Can you work these out from the model? Positions are in its coordinate system, mm. A direction names the side the tool comes from. Give positions to 0.01 mm unless a question says otherwise; leave off trailing zeros. Order: outer loops, then holes, each group sorted by start corner. A loop starts at its lowest first (then second) coordinate and runs counter-clockwise, first axis right, second up. Notation, with made-up numbers: (26, -7.75) - (49, -7.75) arc R26 cw to (49, 10.25) - close; hole circle Ø6 at (3.5, 58). An arc over 180 degrees is marked (long way). Answer as a JSON object with one key per item and string values.
```python
from build123d import *

# Parameters (mm, degrees)
BOSS_EXTRUDE1_DEPTH = 1.27


with BuildPart() as part:
    # Sketch1 → Boss-Extrude1 (new body)
    with BuildSketch(Plane(origin=(0, 0, 0), x_dir=(1, 0, 0), z_dir=(0, 1, 0))):
        with BuildLine():
            Line((-152.4, 120.65), (-139.7, -120.65))
            Line((-139.7, -120.65), (-134.247237287, -224.252491542))
            ThreePointArc((-134.247237287, -224.252491542), (-122.423123118, -249.88969001), (-96.19989799, -260.35))
            Line((-96.19989799, -260.35), (0, -260.35))
            Line((0, -260.35), (96.19989799, -260.35))
            ThreePointArc((96.19989799, -260.35), (122.423123118, -249.88969001), (134.247237287, -224.252491542))
            Line((134.247237287, -224.252491542), (139.7, -120.65))
            Line((139.7, -120.65), (152.4, 120.65))
            Line((152.4, 120.65), (155.939618828, 187.902757734))
            Line((155.939618828, 187.902757734), (79.375, 196.85))
            Line((79.375, 196.85), (66.675, 184.15))
            Line((66.675, 184.15), (0, 184.15))
            Line((0, 184.15), (-66.675, 184.15))
            Line((-66.675, 184.15), (-79.375, 196.85))
            Line((-79.375, 196.85), (-155.939618828, 187.902757734))
            Line((-155.939618828, 187.902757734), (-152.4, 120.65))
        make_face()
        Polygon((-38.1, 95.25), (0, 120.65), (38.1, 95.25), (38.1, -95.25), (0, -120.65), (-38.1, -95.25), align=None, mode=Mode.SUBTRACT)
    extrude(amount=BOSS_EXTRUDE1_DEPTH)


solid = part.part
```
Q1. Which directions (+Z, -Z, +X, -X, +Y, -Y) give clear straight access to the entire face, cutting with the end or side of a thin tool? Please do faces 4 (the face through (18.78, 0.63, -108.13)), 5 (the face through (-72.936, 0.626, -190.411)), 6 (the face through (-122.715, 0.626, 249.609)).
Recorded:
{"face 4": "+Y, -Y", "face 5": "-Z, +Y, -Y", "face 6": "+Z, -X, +Y, -Y"}
Q2. If we section it at B-B, the plane z = -108.5: Please give me the cut outline in (x, y) (3 decimals), then the cut area to 3 significant figures.
Recorded:
{"outline": "(-151.761, 0) - (-18.225, 0) - (-18.225, 1.27) - (-151.761, 1.27) - close; (18.225, 0) - (151.761, 0) - (151.761, 1.27) - (18.225, 1.27) - close", "area": "339 mm^2"}
Q3. If we section it at C-C, the plane z = -49: Please give me the cut outline in (x, y), then the cut area to 3 significant figures.
Recorded:
{"outline": "(-148.63, 0) - (-38.1, 0) - (-38.1, 1.27) - (-148.63, 1.27) - close; (38.1, 0) - (148.63, 0) - (148.63, 1.27) - (38.1, 1.27) - close", "area": "281 mm^2"}
Q4. I need wall thicknesses on L1, parallel to X at y = 0.7, z = -51; L2, parallel to X at y = 0.5, z = -12; L3, parallel to Z at x = 58.5, y = 0.2. Which ranges of each line are inside material? Lowest first, please.
Recorded:
{"L1": "x = -148.73 to -38.1, 38.1 to 148.73", "L2": "x = -146.68 to -38.1, 38.1 to 146.68", "L3": "z = -184.15 to 260.35"}
Q5. We'd pull the mould along X, two halves only. Please class faces 1 (the face through (67, 1.27, 29)), 2 (the face through (122.128, 0.626, 250.167)), 3 (the face through (-19.32, 0.63, -107.77)): released by +X, released by -X, zero draft, split by the parting line, or undercut.
Recorded:
{"face 1": "zero draft", "face 2": "released by +X", "face 3": "undercut"}
Q6. If we section it at D-D, the plane x = 116: Please give me the cut outline in (y, z), then the cut area to 3 significant figures.
Recorded:
{"outline": "(0, -192.57) - (1.27, -192.57) - (1.27, 254.8) - (0, 254.8) - close", "area": "568 mm^2"}
